Here's how the part is built. I have some questions about the finished solid (model axes, mm). A direction names the side the tool comes from. Round coordinates to 2 decimals unless told otherwise and drop trailing zeros. Write each loop counter-clockwise with the first axis right and the second up, starting at its lowest first coordinate (ties: lowest second). Pieces come first, ordered by that corner, then holes. Notation, with made-up numbers: (-24, 19.25) - (3, 19.25) arc R20 cw to (3, 36.25) - close; hole circle Ø5 at (56.5, 46). An arc over 180 degrees is marked (long way). Return JSON: item names as keys, results as strings. Group by question number.
```python
from build123d import *

# Parameters (mm, degrees)
SKETCH1_W           = 57.15
SKETCH1_H           = 88.9
SKETCH1_W_2         = 44.45
SKETCH1_H_2         = 25.4
BOSS_EXTRUDE1_DEPTH = 6.35
SKETCH2_W           = 6.35
SKETCH2_H           = 9.525
SKETCH2_W_2         = 9.525
SKETCH2_H_2         = 6.35
BOSS_EXTRUDE3_DEPTH = 6.35


with BuildPart() as part:
    # Sketch1 → Boss-Extrude1 (new body)
    with BuildSketch(Plane.XY):
        with Locations((28.575, -44.45)):
            Rectangle(SKETCH1_W, SKETCH1_H)
        with Locations((28.575, -69.85)):
            Rectangle(SKETCH1_W_2, SKETCH1_H_2, mode=Mode.SUBTRACT)
    extrude(amount=BOSS_EXTRUDE1_DEPTH)

    # Sketch2 → Boss-Extrude3 (add)
    with BuildSketch(Plane.XY.offset(6.35)):
        with Locations((-3.175, -14.2875)):
            Rectangle(SKETCH2_W, SKETCH2_H)
        with Locations((-3.175, -33.3375)):
            Rectangle(SKETCH2_W, SKETCH2_H)
        with Locations((-3.175, -52.3875)):
            Rectangle(SKETCH2_W, SKETCH2_H)
        with Locations((-3.175, -71.4375)):
            Rectangle(SKETCH2_W, SKETCH2_H)
        with Locations((4.7625, -92.075)):
            Rectangle(SKETCH2_W_2, SKETCH2_H_2)
        with Locations((23.8125, -92.075)):
            Rectangle(SKETCH2_W_2, SKETCH2_H_2)
        with Locations((42.8625, -92.075)):
            Rectangle(SKETCH2_W_2, SKETCH2_H_2)
        with Locations((60.325, -14.2875)):
            Rectangle(SKETCH2_W, SKETCH2_H)
        with Locations((60.325, -33.3375)):
            Rectangle(SKETCH2_W, SKETCH2_H)
        with Locations((60.325, -71.4375)):
            Rectangle(SKETCH2_W, SKETCH2_H)
        with Locations((60.325, -52.3875)):
            Rectangle(SKETCH2_W, SKETCH2_H)
    extrude(amount=-BOSS_EXTRUDE3_DEPTH)


solid = part.part
```
1) Imagine slicing it at A-A (x = 46). Please give me the cut outline in (y, z).
2) Will these pins go through, and if not, where does the flat tip stop? pin 1 Ø3 at (x, z) = (61, 2) entering from -Y; pin 2 Ø1.9 at (y, z) = (-93, 3) entering from +X (3 decimals); pin 3 Ø1.5 at (y, z) = (-41.5, 3) entering from +X.
3) I need wall thicknesses on line 1 along Y through (x, z) = (14.5, 0.5); line 2 along Y through (x, z) = (-2, 3) (3 decimals); line 3 along Y through (x, z) = (20.5, 1). Which ranges of each line are inside material? Lowest first, please.
4) Imagine slicing it at C-C (y = -20). Please give me the cut outline in (x, z).
5) Imagine slicing it at B-B (x = 58.5). Please give me the cut outline in (y, z) (3 decimals), plus the area to 3 significant figures.
6) If we mould it in two halves opening along Y, with no side actions, what happens to faces 1 (the flat face through (63.5, -72, 3)), 2 (the flat face through (60, -19.05, 3)), 3 (the flat face through (5, -95.25, 3))? For each: released by +Y, released by -Y, zero draft, split by the parting line, or undercut.
7) For faces 4 (the flat face through (57.15, -62, 3)), 5 (the flat face through (0, -43, 3)), 6 (the flat face through (0, -86, 3)), which set-ups out of +Z, -Z, +X, -X, +Y, -Y let a thin tool reach every point of the face, with its end or its side?
Results found:
{
 "1": {"outline": "(-95.25, 0) - (-82.55, 0) - (-82.55, 6.35) - (-95.25, 6.35) - close; (-57.15, 0) - (0, 0) - (0, 6.35) - (-57.15, 6.35) - close"},
 "2": {"pin 1": "stops at y = -76.2", "pin 2": "stops at x = 47.625", "pin 3": "stops at x = 57.15"},
 "3": {"line 1": "y = -88.9 to -82.55, -57.15 to 0", "line 2": "y = -76.2 to -66.675, -57.15 to -47.625, -38.1 to -28.575, -19.05 to -9.525", "line 3": "y = -95.25 to -82.55, -57.15 to 0"},
 "4": {"outline": "(0, 0) - (57.15, 0) - (57.15, 6.35) - (0, 6.35) - close"},
 "5": {"outline": "(-76.2, 0) - (-66.675, 0) - (-66.675, 6.35) - (-76.2, 6.35) - close; (-57.15, 0) - (-47.625, 0) - (-47.625, 6.35) - (-57.15, 6.35) - close; (-38.1, 0) - (-28.575, 0) - (-28.575, 6.35) - (-38.1, 6.35) - close; (-19.05, 0) - (-9.525, 0) - (-9.525, 6.35) - (-19.05, 6.35) - close", "area": "242 mm²"},
 "6": {"face 1": "zero draft", "face 2": "undercut", "face 3": "released by -Y"},
 "7": {"face 4": "+Z, -Z, +X", "face 5": "+Z, -Z, -X", "face 6": "+Z, -Z, -X, -Y"}
}
